Input: part model. Units: mm. Frame: model coordinates. A direction names the side the tool comes from. Round coordinates to 2 decimals unless told otherwise and drop trailing zeros. Loops run counter-clockwise (first coordinate to the right, second up) from the corner with the lowest first, then second, coordinate; pieces in that order, holes last. Notation, with made-up numbers: M 18,19 L 74,19 A25 cw 74,39 Z; hole C -27.5,-37.5 d3. An arc over 180 degrees is marked long. Use one line per item in the form item = value. Start each with the question number.
Q1. First-contact query: P1, Ø1.9, axis at y = 1.5, z = 36, coming from the +X side (3 decimals); P2, Ø1.4, axis at y = 3.18, z = 35.17, coming from the +X side; P3, Ø2, axis at y = 5.5, z = -3.5, coming from the -X side. Flat tips, straight axial feed; report the tip coordinate or a pass-through.
Q2. Mould query, pull axis Y, two halves, no side actions, for faces 3 (the flat face through (0, 0, 3)), 4 (the cylindrical face through (7.875, 3.126, 30.503)), 5 (the flat face through (0, 6.35, 3)). Classes: pulls with the +Y half, pulls with the -Y half, needs draft (parallel to the pull), parting line crosses it, or undercut.
Q3. Ray query, line 1 along Y through (x, z) = (5.5, 31); line 2 along X through (y, z) = (5, 30.5); line 3 along X through (y, z) = (2, -18). Return the intervals inside material, ascending.
Q4. Access query for faces 1 (the cylindrical face through (-7.875, 3.224, 30.503)), 2 (the flat face through (0, 3, -31.75)). Directions: +Z, -Z, +X, -X, +Y, -Y. A direction counts if a zero-diameter tool reaches every point of the face in a straight line with its end or side. Return the directions, or none.
Q5. Section query A-A, the plane x = -8. Output: boundary loops of the cut face in (y, z) (3 decimals), and give its area (3 significant figures).
Q6. Section query B-B, the plane z = 33.5. Output: boundary loops of the cut face in (x, y) (3 decimals).
```python
from build123d import *

# Parameters (mm, degrees)
SKETCH1_RX               = 38.1
SKETCH1_RY               = 21.209
BOSS_EXTRUDE1_DEPTH      = 6.35
CUT_EXTRUDE6_DEPTH       = 45.065339906
SKETCH35_W               = 18.034
SKETCH35_H               = 6.35
CUT_EXTRUDE17_DEPTH      = 45.065339906
SKETCH36_R               = 0.762
CUT_EXTRUDE18_DEPTH      = 46.678353405
SKETCH37_R               = 4.664778091
CUT_EXTRUDE19_DEPTH      = 46.678353405
SKETCH38_R               = 4.664778091
CUT_EXTRUDE20_DEPTH      = 46.678353405
CUT_EXTRUDE21_DEPTH      = 46.678353405
CUT_EXTRUDE21_DEPTH_BACK = 46.678353405
SKETCH39_W               = 2.364149351
SKETCH39_H               = 6.35
BOSS_EXTRUDE2_DEPTH      = 6.35
CUT_EXTRUDE22_DEPTH      = 46.029039702
CUT_EXTRUDE22_DEPTH_BACK = 46.029039702


with BuildPart() as part:
    # Sketch1 → Boss-Extrude1 (new body)
    with BuildSketch(Plane(origin=(0, 0, 0), x_dir=(1, 0, 0), z_dir=(0, 1, 0))):
        with Locations(Location((0, 0), (0, 0, 90))):
            Ellipse(SKETCH1_RX, SKETCH1_RY)
    extrude(amount=BOSS_EXTRUDE1_DEPTH)

    # Sketch7 → Cut-Extrude6 (cut, through all)
    with BuildSketch(Plane(origin=(0, 6.35, 0), x_dir=(1, 0, 0), z_dir=(0, 1, 0))):
        with BuildLine():
            Line((-11.723715863, 31.75), (11.723715863, 31.75))
            add(Edge.make_bspline(
                [(11.723715863, 31.75), (0, 45.72), (-11.723715863, 31.75)],
                knots=[5.697499764, 5.697499764, 5.697499764, 6.868870851, 6.868870851, 6.868870851], degree=2, weights=[1, 0.833333333, 1]))
        make_face()
    extrude(amount=-CUT_EXTRUDE6_DEPTH, mode=Mode.SUBTRACT)

    # Sketch35 → Cut-Extrude17 (cut, through all)
    with BuildSketch(Plane(origin=(0, 6.35, 0), x_dir=(1, 0, 0), z_dir=(0, 1, 0))):
        with Locations((12.192, -34.925)):
            Rectangle(SKETCH35_W, SKETCH35_H)
        with Locations((-12.192, -34.925)):
            Rectangle(SKETCH35_W, SKETCH35_H)
    extrude(amount=-CUT_EXTRUDE17_DEPTH, mode=Mode.SUBTRACT)

    # Sketch36 → Cut-Extrude18 (cut, through all)
    with BuildSketch(Plane.ZY.offset(3.175)):
        with Locations((35.167532682, 3.175)):
            Circle(SKETCH36_R)
    extrude(amount=-CUT_EXTRUDE18_DEPTH, mode=Mode.SUBTRACT)

    # Sketch37 → Cut-Extrude19 (cut, through all)
    with BuildSketch(Plane.ZY.offset(3.175)):
        with Locations((35.167532682, 3.175)):
            Circle(SKETCH37_R)
    extrude(amount=CUT_EXTRUDE19_DEPTH, mode=Mode.SUBTRACT)

    # Sketch38 → Cut-Extrude20 (cut, through all)
    with BuildSketch(Plane(origin=(3.175, 0, 0), x_dir=(0, 0, -1), z_dir=(1, 0, 0))):
        with Locations((-35.167532682, 3.175)):
            Circle(SKETCH38_R)
    extrude(amount=CUT_EXTRUDE20_DEPTH, mode=Mode.SUBTRACT)

    # Sketch39 → Cut-Extrude21 (cut, two sides: drawn at the far end of the back side and taken through both)
    with BuildSketch(Plane.ZY.offset(3.175).offset(-CUT_EXTRUDE21_DEPTH_BACK)):
        with Locations((38.852740041, 3.175)):
            Rectangle(SKETCH39_W, SKETCH39_H)
    extrude(amount=CUT_EXTRUDE21_DEPTH + CUT_EXTRUDE21_DEPTH_BACK, mode=Mode.SUBTRACT)

    # Sketch40 → Boss-Extrude2 (add)
    with BuildSketch(Plane.ZY.offset(3.175)):
        with BuildLine():
            Line((37.670665365, 6.35), (37.670665365, 0))
            ThreePointArc((37.670665365, 0), (39.210588238, 3.175), (37.670665365, 6.35))
        make_face()
    extrude(amount=-BOSS_EXTRUDE2_DEPTH)

    # Sketch41 → Cut-Extrude22 (cut, two sides: drawn at the far end of the back side and taken through both)
    with BuildSketch(Plane(origin=(0, 0, 0), x_dir=(0, 0, -1), z_dir=(1, 0, 0)).offset(-CUT_EXTRUDE22_DEPTH_BACK)):
        Polygon((-35.808924316, 0), (-40.546826373, 1.914236687), (-40.546826373, -0.644343838), (-35.808924316, -0.644343838), align=None)
    extrude(amount=CUT_EXTRUDE22_DEPTH + CUT_EXTRUDE22_DEPTH_BACK, mode=Mode.SUBTRACT)


solid = part.part
```
Results found:
q1.P1 = 3.175
q1.P2 = through
q1.P3 = -21.16
q2.face_3 = pulls with the -Y half
q2.face_4 = undercut
q2.face_5 = pulls with the +Y half
q3.line_1 = 0 to 1.08, 5.27 to 6.35
q3.line_2 = -12.71 to 12.71
q3.line_3 = -18.69 to 18.69
q4.face_1 = +Z, -X
q4.face_2 = -Z, +X, -X, +Y, -Y
q5.outline = M 0,-31.75 L 6.35,-31.75 L 6.35,31.75 A4.665 cw 0,31.75 Z
q5.area = 398 mm²
q6.outline = M -3.175,0 L 3.175,0 L 3.175,6.35 L -3.175,6.35 Z
